Job drawing, mm, ordinate dimensions from the low corner. One solid piece. A direction names the side the tool comes from. Give positions to 0.01 mm unless a question says otherwise; leave off trailing zeros. Order: outer loops, then holes, each group sorted by start corner. A loop starts at its lowest first (then second) coordinate and runs counter-clockwise, first axis right, second up. Notation, with made-up numbers: M 72,37 L 115,37 A19 ccw 115,66 Z; hole C 2.25,21.5 d2. An arc over 180 degrees is marked long. Use CSV: the item, a comma, the result in double quotes. Start each with the question number.
Item 1: Band-saw the part on D-D on y = 21. Write the cut outline in (x, z).
Item 2: Which spindle directions (+Z, -Z, +X, -X, +Y, -Y) get a long thin tool onto all of the face, cutting with end or side? Do the marked faces 4 and 5. Say none if no direction does.
Item 3: Band-saw the part on C-C on x = 2.5. Write the cut outline in (y, z) (1 decimal).
Item 4: Two-plate mould, pull along Y, no slides. Class the marked faces 1, 2 and 3: pulls with the +Y half, pulls with the -Y half, needs draft (parallel to the pull), parting line crosses it, or undercut.
Item 5: Band-saw the part on B-B on y = 25. Write the cut outline in (x, z).
Item 6: Wall check: line 1 along Y through (x, z) = (1, 41.5) (1 decimal); line 2 along Y through (x, z) = (2.5, 19.5) (1 decimal); line 3 along Z through (x, y) = (2, 25.5). Give the ranges that are in metal, low to high.
Item 7: Pin check, flat tips, straight feed: P1, Ø10, axis at y = 34.5, z = 38, coming from the -X side; P2, Ø4, axis at y = 10.5, z = 28.5, coming from the -X side. Stop position of each tip, or through.
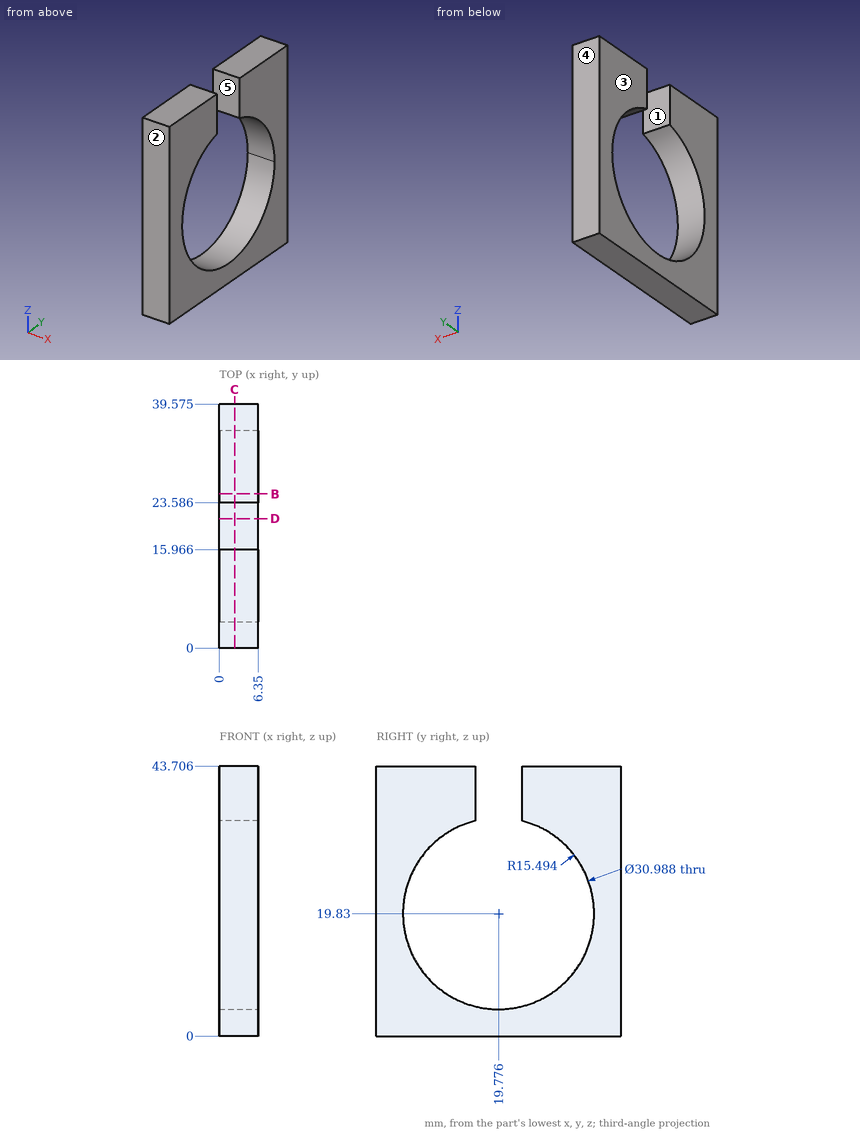
Model answer:
1,outline,"M 0,0 L 6.35,0 L 6.35,4.38 L 0,4.38 Z"
2,face 4,"+Z, -Z, +X, -X, +Y"
2,face 5,"+Z, +X, -X"
3,outline,"M 0,0 L 39.6,0 L 39.6,43.7 L 23.6,43.7 L 23.6,34.8 A15.5 cw long 16,34.8 L 16,43.7 L 0,43.7 Z"
4,face 1,"undercut"
4,face 2,"pulls with the -Y half"
4,face 3,"needs draft"
5,outline,"M 0,0 L 6.35,0 L 6.35,5.24 L 0,5.24 Z; M 0,34.42 L 6.35,34.42 L 6.35,43.71 L 0,43.71 Z"
6,line 1,"y = 0 to 16, 23.6 to 39.6"
6,line 2,"y = 0 to 4.3, 35.3 to 39.6"
6,line 3,"z = 0 to 5.43, 34.23 to 43.71"
7,P1,"stops at x = 0"
7,P2,"passes through"
